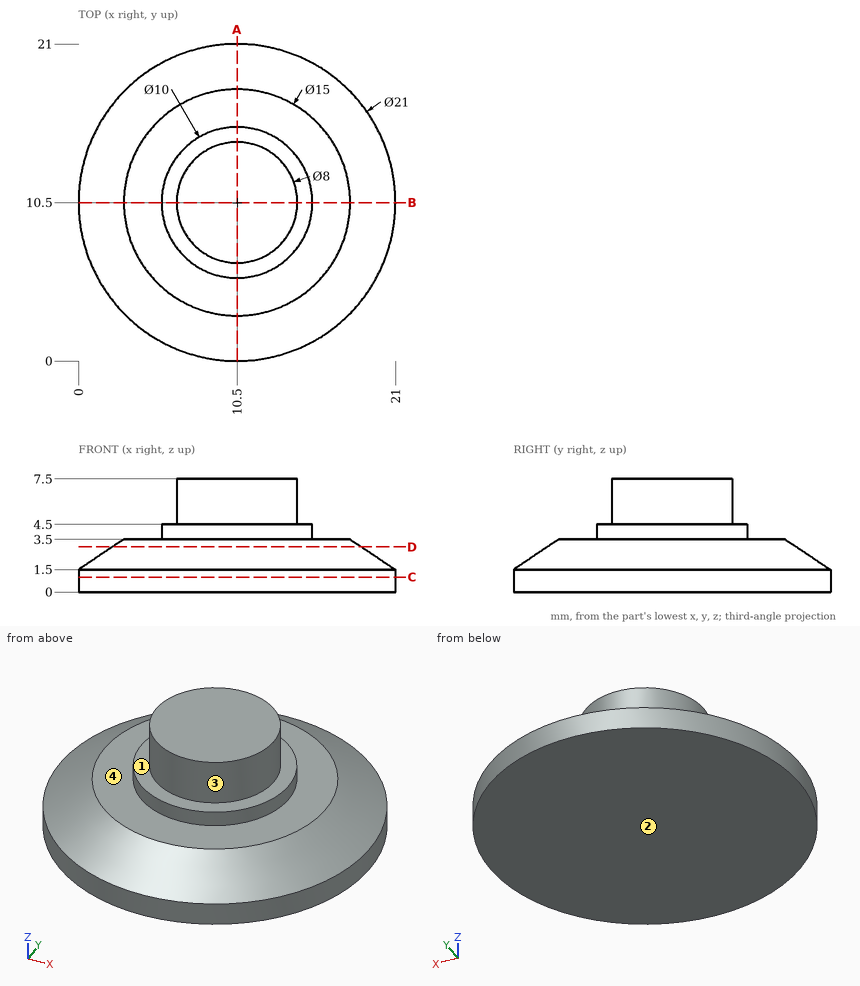
Can you work these out from the drawing? Everything is in mm from the part's minimum corner. A direction names the side the tool comes from. Give positions to 0.01 mm unless a question says otherwise; leave off trailing zeros. Order: outer loops, then holes, each group sorted by start corner. A loop starts at its lowest first (then second) coordinate and runs counter-clockwise, first axis right, second up.
1. For the marked faces 1 and 2, which set-ups out of +Z, -Z, +X, -X, +Y, -Y let a thin tool reach every point of the face, with its end or its side?
2. Suppose I cut it at C-C (z = 1). List the corners of the cut face in (x, y) for me, plus the area to 3 significant figures.
3. I need wall thicknesses on L1, parallel to Z at x = 6, y = 11; L2, parallel to Z at x = 4.5, y = 11.5; L3, parallel to Y at x = 11.75, z = 0.5. Which ranges of each line are inside material? Lowest first, please.
4. Suppose I cut it at D-D (z = 3). List the corners of the cut face in (x, y) for me.
5. Will these pins go through, and if not, where does the flat tip stop? P1, Ø1, axis at x = 11.5, z = 3.5, coming from the +Y side; P2, Ø8, axis at x = 17, y = 17, coming from the +Z side.
6. Suppose I cut it at A-A (x = 10.5). List the corners of the cut face in (y, z) for me.
7. We'd pull the mould along X, two halves only. Please class the marked faces 3 and 4: pulls with the +X half, pulls with the -X half, needs draft (parallel to the pull), parting line crosses it, or undercut.
Solved:
1. face 1: +Z
1. face 2: -Z, +X, -X, +Y, -Y
2. outline: circle Ø21 at (10.5, 10.5)
2. area: 346 mm2
3. L1: z = 0 to 4.5
3. L2: z = 0 to 3.5
3. L3: y = 0.07 to 20.93
4. outline: circle Ø16.5 at (10.5, 10.5)
5. P1: stops at y = 18.69
5. P2: stops at z = 3.5
6. outline: (0, 0) - (21, 0) - (21, 1.5) - (18, 3.5) - (15.5, 3.5) - (15.5, 4.5) - (14.5, 4.5) - (14.5, 7.5) - (6.5, 7.5) - (6.5, 4.5) - (5.5, 4.5) - (5.5, 3.5) - (3, 3.5) - (0, 1.5) - close
7. face 3: parting line crosses it
7. face 4: needs draft
